Input: part model. Units: mm. Frame: model coordinates. A direction names the side the tool comes from. Coordinates: 2 decimals unless noted, no trailing zeros. Loops run counter-clockwise (first coordinate to the right, second up) from the corner with the lowest first, then second, coordinate; pieces in that order, holes last.
Item 1: Section C-C on z = 4.5. Return loops of the section in (x, y).
Item 2: Section B-B on x = 0. Return loops of the section in (y, z).
Item 3: Section A-A on y = 0. Return loops of the section in (x, z) (3 decimals), and give its area (3 significant figures).
Item 4: Ray query, line 1 along X through (y, z) = (-3, 13.75); line 2 along Y through (x, z) = (-17, 15); line 3 along Y through (x, z) = (27, 25.25). Return the intervals inside material, ascending.
Item 5: Section D-D on x = 21. Return loops of the section in (y, z).
Item 6: Contact query for flat-ended pins moving along their axis: P1, Ø5, axis at y = -3, z = 17.5, coming from the +X side; P2, Ø23, axis at x = 1.5, y = 3.5, coming from the +Z side; P3, Ø1, axis at x = -24.71, z = 21.675, coming from the -Y side; P4, Ø3, axis at y = -7, z = 23, coming from the -X side. Output: stop coordinate, or through.
Item 7: Reachability of faces 1 (the flat face through (-20.25, -2, 17)), 2 (the flat face through (-24, -10.5, 17)), 3 (the cylindrical face through (3.54, 23.96, 7.33)), 4 (the flat face through (-20.25, 19, 17)), 5 (the cylindrical face through (10, 3.2, 4.3)) from +Z, -Z, +X, -X, +Y, -Y: full face, straight path, thin tool, end or side. Return the list, or none.
Item 8: Pull-direction query (Y, two-part tool) for faces 6 (the flat face through (2, 26.5, 16)), 7 (the cylindrical face through (-0.59, 4.46, 0.42)), 8 (the flat face through (0, -21, 3)), 9 (the flat face through (27.5, -2, 17)); classes: released by +Y, released by -Y, zero draft, split by the parting line, or undercut.
```python
from build123d import *

# Parameters (mm, degrees)
ESQUISSE1_W              = 55
ESQUISSE1_H              = 43
BOSS_EXTRU_1_DEPTH       = 27
ESQUISSE2_W              = 40.5
ESQUISSE2_H              = 21.676575317
ENL_V_MAT_EXTRU_1_DEPTH  = 38
ESQUISSE3_R              = 0.7
ENL_V_MAT_EXTRU_2_DEPTH  = 43
ESQUISSE4_W              = 55
ESQUISSE4_H              = 20.5
ENL_V_MAT_EXTRU_3_DEPTH  = 11
ENL_V_MAT_EXTRU_6_REACH  = 66.933
ESQUISSE5_W              = 20.5
ESQUISSE5_H              = 10
ESQUISSE6_W              = 7.25
ESQUISSE6_H              = 20.5
ENL_V_MAT_EXTRU_7_DEPTH  = 5
ESQUISSE7_R              = 31
BOSS_EXTRU_2_DEPTH       = 6.5
ESQUISSE8_R              = 41
ESQUISSE8_R_2            = 31
ENL_V_MAT_EXTRU_8_DEPTH  = 6.5
TROU_TARAUD_M2X0_41_D    = 1.6
ESQUISSE10_R             = 10.5
ENL_V_MAT_EXTRU_9_DEPTH  = 4.5
ESQUISSE11_R             = 4.5
ENL_V_MAT_EXTRU_10_DEPTH = 2
ESQUISSE12_R             = 9.25
ESQUISSE12_R_2           = 1.25
BOSS_EXTRU_3_DEPTH       = 5
ESQUISSE13_W             = 50.114904395
ESQUISSE13_H             = 12.012600019
ENL_V_MAT_EXTRU_11_DEPTH = 6.5
BOSS_EXTRU_4_START       = 1.2
BOSS_EXTRU_4_DEPTH       = 1.2
ESQUISSE15_W             = 53.005482756
ESQUISSE15_H             = 10
ENL_V_MAT_EXTRU_12_DEPTH = 7.7
ESQUISSE16_R             = 4.5
ENL_V_MAT_EXTRU_13_DEPTH = 1.2


with BuildPart() as part:
    # Esquisse1 → Boss.-Extru.1 (new body)
    with BuildSketch(Plane.XY):
        Rectangle(ESQUISSE1_W, ESQUISSE1_H)
    extrude(amount=BOSS_EXTRU_1_DEPTH)

    # Esquisse2 → Enlèv. mat.-Extru.1 (cut)
    with BuildSketch(Plane.XZ.offset(21.5)):
        with Locations((0, 17.338287659)):
            Rectangle(ESQUISSE2_W, ESQUISSE2_H)
    extrude(amount=-ENL_V_MAT_EXTRU_1_DEPTH, mode=Mode.SUBTRACT)

    # Esquisse3 → Enlèv. mat.-Extru.2 (cut)
    with BuildSketch(Plane.XZ.offset(21.5)):
        with Locations(Location((-24.71, 21.675, 0), (0, 0, 270))):
            Circle(ESQUISSE3_R)
        with Locations(Location((-24.71, 11.825, 0), (0, 0, 270))):
            Circle(ESQUISSE3_R)
        with Locations(Location((24.71, 11.825, 0), (0, 0, 270))):
            Circle(ESQUISSE3_R)
        with Locations(Location((24.71, 21.675, 0), (0, 0, 270))):
            Circle(ESQUISSE3_R)
    extrude(amount=-ENL_V_MAT_EXTRU_2_DEPTH, mode=Mode.SUBTRACT)

    # Esquisse4 → Enlèv. mat.-Extru.3 (cut)
    with BuildSketch(Plane.XZ.offset(21.5)):
        with Locations((0, 16.75)):
            Rectangle(ESQUISSE4_W, ESQUISSE4_H)
    extrude(amount=-ENL_V_MAT_EXTRU_3_DEPTH, mode=Mode.SUBTRACT)

    # Enlèv. mat.-Extru.6: up to this face of the body (flat: up to its plane)
    enl_v_mat_extru_6_end = Plane(part.part.faces().sort_by_distance((27.5, 3.85676109, 12.716595404))[0])
    # Esquisse5 → Enlèv. mat.-Extru.6 (cut, up to the picked face)
    with BuildSketch(Plane.ZY.offset(27.5), mode=Mode.PRIVATE) as enl_v_mat_extru_6_sk1:
        with Locations((16.75, 11.5)):
            Rectangle(ESQUISSE5_W, ESQUISSE5_H)
    enl_v_mat_extru_6_tool1 = split(extrude(enl_v_mat_extru_6_sk1.sketch, amount=-ENL_V_MAT_EXTRU_6_REACH, mode=Mode.PRIVATE), bisect_by=enl_v_mat_extru_6_end, keep=Keep.BOTH, mode=Mode.PRIVATE)
    add(enl_v_mat_extru_6_tool1.solids().sort_by(Axis((-27.5, 11.5, 16.75), (1, 0, 0)))[0], mode=Mode.SUBTRACT)

    # Esquisse6 → Enlèv. mat.-Extru.7 (cut)
    with BuildSketch(Plane.XZ.offset(-16.5)):
        with Locations((-23.875, 16.75)):
            Rectangle(ESQUISSE6_W, ESQUISSE6_H)
        with Locations((23.875, 16.75)):
            Rectangle(ESQUISSE6_W, ESQUISSE6_H)
    extrude(amount=-ENL_V_MAT_EXTRU_7_DEPTH, mode=Mode.SUBTRACT)

    # Esquisse7 → Boss.-Extru.2 (add)
    with BuildSketch(Plane(origin=(0, 0, 0), x_dir=(-1, 0, 0), z_dir=(0, 0, -1))):
        Circle(ESQUISSE7_R)
    extrude(amount=-BOSS_EXTRU_2_DEPTH)

    # Esquisse8 → Enlèv. mat.-Extru.8 (cut)
    with BuildSketch(Plane(origin=(0, 0, 0), x_dir=(-1, 0, 0), z_dir=(0, 0, -1))):
        Circle(ESQUISSE8_R)
        Circle(ESQUISSE8_R_2, mode=Mode.SUBTRACT)
    extrude(amount=-ENL_V_MAT_EXTRU_8_DEPTH, mode=Mode.SUBTRACT)

    # Trou taraudé M2x0.41 (through all)
    with Locations(Plane(origin=(-24.71, -10.5, 21.675), x_dir=(0, 0, -1), z_dir=(0, -1, 0))):
        with Locations((0, 0), (9.85, 0), (0, 49.42), (9.85, 49.42)):
            Hole(TROU_TARAUD_M2X0_41_D / 2)

    # Esquisse10 → Enlèv. mat.-Extru.9 (cut)
    with BuildSketch(Plane.XY.offset(6.5)):
        Circle(ESQUISSE10_R)
    extrude(amount=-ENL_V_MAT_EXTRU_9_DEPTH, mode=Mode.SUBTRACT)

    # Esquisse11 → Enlèv. mat.-Extru.10 (cut)
    with BuildSketch(Plane.XY.offset(2)):
        Circle(ESQUISSE11_R)
    extrude(amount=-ENL_V_MAT_EXTRU_10_DEPTH, mode=Mode.SUBTRACT)

    # Esquisse12 → Boss.-Extru.3 (add)
    with BuildSketch(Plane(origin=(0, 21.5, 0), x_dir=(1, 0, 0), z_dir=(0, 1, 0))):
        with Locations(Location((0, -15.876822983, 0), (0, 0, 90))):
            Circle(ESQUISSE12_R)
        with Locations(Location((0, -15.876822983, 0), (0, 0, 270))):
            Circle(ESQUISSE12_R_2, mode=Mode.SUBTRACT)
    extrude(amount=BOSS_EXTRU_3_DEPTH)

    # Esquisse13 → Enlèv. mat.-Extru.11 (cut)
    with BuildSketch(Plane.XY.offset(6.5)):
        with Locations((-0.983340997, 27.50630001)):
            Rectangle(ESQUISSE13_W, ESQUISSE13_H)
    extrude(amount=-ENL_V_MAT_EXTRU_11_DEPTH, mode=Mode.SUBTRACT)

    # Esquisse14 → Boss.-Extru.4 (add)
    with BuildSketch(Plane(origin=(0, 0, 0), x_dir=(-1, 0, 0), z_dir=(0, 0, -1)).offset(BOSS_EXTRU_4_START)):
        with BuildLine():
            Line((-22.332711434, 21.5), (22.332711434, 21.5))
            ThreePointArc((22.332711434, 21.5), (0, -31), (-22.332711434, 21.5))
        make_face()
    extrude(amount=-BOSS_EXTRU_4_DEPTH)

    # Esquisse15 → Enlèv. mat.-Extru.12 (cut)
    with BuildSketch(Plane.XY.offset(6.5)):
        with Locations((0, -26)):
            Rectangle(ESQUISSE15_W, ESQUISSE15_H)
    extrude(amount=-ENL_V_MAT_EXTRU_12_DEPTH, mode=Mode.SUBTRACT)

    # Esquisse16 → Enlèv. mat.-Extru.13 (cut)
    with BuildSketch(Plane.XY):
        Circle(ESQUISSE16_R)
    extrude(amount=-ENL_V_MAT_EXTRU_13_DEPTH, mode=Mode.SUBTRACT)


solid = part.part
```
Results found:
1. outline: (-22.8, -21) - (22.8, -21) arc R31 ccw to (22.33, 21.5) - (-22.33, 21.5) arc R31 ccw to start; hole circle Ø21 at (0, 0)
2. outline: (-21, -1.2) - (-4.5, -1.2) - (-4.5, 2) - (-10.5, 2) - (-10.5, 6.5) - (-21, 6.5) - close; (4.5, -1.2) - (21.5, -1.2) - (21.5, 6.63) - (26.5, 6.63) - (26.5, 14.63) - (21.5, 14.63) - (21.5, 17.13) - (26.5, 17.13) - (26.5, 25.13) - (21.5, 25.13) - (21.5, 27) - (16.5, 27) - (16.5, 6.5) - (10.5, 6.5) - (10.5, 2) - (4.5, 2) - close
3. outline: (-31, -1.2) - (-4.5, -1.2) - (-4.5, 2) - (-10.5, 2) - (-10.5, 6.5) - (-20.25, 6.5) - (-20.25, 27) - (-27.5, 27) - (-27.5, 6.5) - (-31, 6.5) - close; (4.5, -1.2) - (31, -1.2) - (31, 6.5) - (27.5, 6.5) - (27.5, 27) - (20.25, 27) - (20.25, 6.5) - (10.5, 6.5) - (10.5, 2) - (4.5, 2) - close; hole circle Ø1.6 at (-24.71, 11.825); hole circle Ø1.6 at (-24.71, 21.675); hole circle Ø1.6 at (24.71, 11.825); hole circle Ø1.6 at (24.71, 21.675)
3. area: 643 mm2
4. line 1: x = -27.5 to -20.25, 20.25 to 27.5
4. line 2: y = 16.5 to 21.5
4. line 3: y = -10.5 to 6.5
5. outline: (-21, -1.2) - (21.5, -1.2) - (21.5, 6.5) - (6.5, 6.5) - (6.5, 27) - (-10.5, 27) - (-10.5, 6.5) - (-21, 6.5) - close
6. P1: stops at x = 27.5
6. P2: stops at z = 6.5
6. P3: passes through
6. P4: stops at x = -27.5
7. face 1: +Z, -Y
7. face 2: +Z, +X, -X, -Y
7. face 3: +Y
7. face 4: +Z, -X, +Y
7. face 5: +Z
8. face 6: released by +Y
8. face 7: undercut
8. face 8: released by -Y
8. face 9: zero draft
